```python
from build123d import *

# Parameters (mm, degrees)
SKETCH1_R           = 3
SKETCH1_R_2         = 1
BOSS_EXTRUDE1_DEPTH = 1.5
SKETCH2_R           = 2.5
SKETCH2_R_2         = 1.5
CUT_EXTRUDE1_DEPTH  = 0.2
CUT_EXTRUDE2_START  = -2.8
SKETCH2_2_R         = 2.5
SKETCH2_2_R_2       = 1.5
CUT_EXTRUDE2_DEPTH  = 0.2


with BuildPart() as part:
    # Sketch1 → Boss-Extrude1 (new, symmetric)
    with BuildSketch(Plane.XY):
        Circle(SKETCH1_R)
        Circle(SKETCH1_R_2, mode=Mode.SUBTRACT)
    extrude(amount=BOSS_EXTRUDE1_DEPTH, both=True)

    # Sketch2 → Cut-Extrude1 (cut)
    with BuildSketch(Plane.XY.offset(1.5)):
        Circle(SKETCH2_R)
        Circle(SKETCH2_R_2, mode=Mode.SUBTRACT)
    extrude(amount=-CUT_EXTRUDE1_DEPTH, mode=Mode.SUBTRACT)

    # Sketch2<2> → Cut-Extrude2 (cut)
    with BuildSketch(Plane.XY.offset(1.5).offset(CUT_EXTRUDE2_START)):
        Circle(SKETCH2_2_R)
        Circle(SKETCH2_2_R_2, mode=Mode.SUBTRACT)
    extrude(amount=-CUT_EXTRUDE2_DEPTH, mode=Mode.SUBTRACT)


solid = part.part
```
Here's how the part is built. I have some questions about the finished solid (model axes, mm). A direction names the side the tool comes from. Coordinates: 2 decimals unless noted, no trailing zeros. Loops run counter-clockwise (first coordinate to the right, second up) from the corner with the lowest first, then second, coordinate; pieces in that order, holes last. Notation, with made-up numbers: (57.5, 6.5) - (89.5, 6.5) arc R24 cw to (89.5, 26.5) - close; hole circle Ø5 at (85.5, -30.5). An arc over 180 degrees is marked (long way). Return JSON: item names as keys, results as strings. Group by question number.
Item 1: We'd pull the mould along X, two halves only. Please class faces 1 (the face through (-3, 0, 0)), 2 (the face through (0, -2, -1.3)), 3 (the face through (-2, 2, -1.5)): +X half, -X half, draft (parallel to the pull), parting line (faces both ways), or undercut.
Item 2: I need wall thicknesses on line 1 (Y direction, x = 0, z = 1.45); line 2 (Y direction, x = 0, z = -0.2); line 3 (Z direction, x = -1.8, y = 1.3). Which ranges of each line are inside material? Lowest first, please. Write a range as from..to.
Item 3: If we section it at D-D on y = -1.4: Write out the boundary of the cut face in (x, z), and give its area (3 significant figures).
Item 4: On a 3-axis mill with a long thin cutter (end or side, diameter ignored), from which of +Z, -Z, +X, -X, +Y, -Y can I reach the whole of each face in a straight line? I mean faces 4 (the face through (0, -1, 0)), 5 (the face through (0, -2, 1.3)). Say none if no direction works.
Item 5: If we section it at A-A on x = 0: Write out the boundary of the cut face in (y, z).
Item 6: If we section it at C-C on z = 0.05: Write out the boundary of the cut face in (x, y).
Calculated:
{
 "1": {"face 1": "parting line", "face 2": "undercut", "face 3": "draft"},
 "2": {"line 1": "y = -3..-2.5, -1.5..-1, 1..1.5, 2.5..3", "line 2": "y = -3..-1, 1..3", "line 3": "z = -1.3..1.3"},
 "3": {"outline": "(-2.65, -1.5) - (-2.07, -1.5) - (-2.07, -1.3) - (-0.54, -1.3) - (-0.54, -1.5) - (0.54, -1.5) - (0.54, -1.3) - (2.07, -1.3) - (2.07, -1.5) - (2.65, -1.5) - (2.65, 1.5) - (2.07, 1.5) - (2.07, 1.3) - (0.54, 1.3) - (0.54, 1.5) - (-0.54, 1.5) - (-0.54, 1.3) - (-2.07, 1.3) - (-2.07, 1.5) - (-2.65, 1.5) - close", "area": "14.7 mm^2"},
 "4": {"face 4": "+Z, -Z", "face 5": "+Z"},
 "5": {"outline": "(-3, -1.5) - (-2.5, -1.5) - (-2.5, -1.3) - (-1.5, -1.3) - (-1.5, -1.5) - (-1, -1.5) - (-1, 1.5) - (-1.5, 1.5) - (-1.5, 1.3) - (-2.5, 1.3) - (-2.5, 1.5) - (-3, 1.5) - close; (1, -1.5) - (1.5, -1.5) - (1.5, -1.3) - (2.5, -1.3) - (2.5, -1.5) - (3, -1.5) - (3, 1.5) - (2.5, 1.5) - (2.5, 1.3) - (1.5, 1.3) - (1.5, 1.5) - (1, 1.5) - close"},
 "6": {"outline": "circle Ø6 at (0, 0); hole circle Ø2 at (0, 0)"}
}
